Geometry check sheet. Reference: the model listing, model coordinates, mm. Face numbers are marked on the shaded views. A direction names the side the tool comes from. Give positions to 0.01 mm unless a question says otherwise; leave off trailing zeros. Order: outer loops, then holes, each group sorted by start corner. A loop starts at its lowest first (then second) coordinate and runs counter-clockwise, first axis right, second up. Notation, with made-up numbers: M 42,36.25 L 80,36.25 A24 cw 80,55.25 Z; hole C 28.5,-26 d3. An arc over 180 degrees is marked long. Put each result on its own line as item: value. Start each with the question number.
Q1. Material ranges on L1, parallel to X at y = -8.5, z = 19.5; L2, parallel to Z at x = -42, y = -15; L3, parallel to X at y = -1.5, z = 32.5, recorded low to high.
Q2. Section check A-A on z = 29.5. Record the cut outline in (x, y), then the cut area to 3 significant figures.
Q3. Go/stop test with flat-tipped pins: pin 1 (1 mm diameter, centred on x = -24.5, z = 7.5, fed in from +Y); pin 2 (11.5 mm diameter, centred on x = -35.5, z = 32.5, fed in from -Y); pin 3 (1.5 mm diameter, centred on x = -23.5, y = -32.5, fed in from +Z); pin 4 (19 mm diameter, centred on x = -27, y = -14.5, fed in from +Z). Record where each tip stops, or that it passes through.
Q4. Section check D-D on y = -21. Record the cut outline in (x, z).
Q5. Access from +Z, -Z, +X, -X, +Y, -Y to the whole of each face (thin tool, end or side, straight path). Record for the marked faces 1, 2 and 3.
Q6. Section check C-C on z = 14.5. Record the cut outline in (x, y).
Q7. Section check B-B on x = -10. Record the cut outline in (y, z), then the cut area to 3 significant figures.
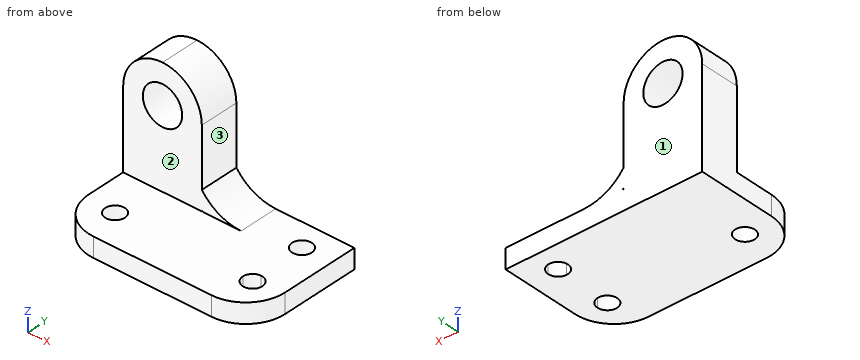
```python
from build123d import *

# Parameters (mm, degrees)
F1_DEPTH  = 38.1
F2_W      = 25.4
F2_H      = 38.1
F3_DEPTH  = 25.4
F4_R      = 6.35
F5_DEPTH  = 12.7
F7_DEPTH  = 6.35
F6_R      = 3.175
F8_DEPTH  = 6.35
F10_DEPTH = 12.7


with BuildPart() as f1:
    # F0 (on Front) → F1 (new body)
    with BuildSketch(Plane.XZ):
        Polygon((-37.0136184096, 45.1297735606), (-62.4136184096, 45.1297735606), (-62.4136184096, 0.6797735606), (1.0863815904, 0.6797735606), (1.0863815904, 7.0297735606), (-37.0136184096, 7.0297735606), align=None)
    extrude(amount=F1_DEPTH)

    # F2 (on face) → F3 (cut)
    with BuildSketch(Plane.XZ.offset(38.1)):
        with Locations((-49.7136184096, 26.0797735606)):
            Rectangle(F2_W, F2_H)
    extrude(amount=-F3_DEPTH, mode=Mode.SUBTRACT)

    # F4 (on face) → F5 (cut)
    with BuildSketch(Plane.XZ.offset(12.7)):
        with BuildLine():
            Line((-62.4136184096, 45.1297735606), (-62.4136184096, 32.4297735606))
            ThreePointArc((-62.4136184096, 32.4297735606), (-58.6938745306, 41.4100296816), (-49.7136184096, 45.1297735606))
            Line((-49.7136184096, 45.1297735606), (-62.4136184096, 45.1297735606))
        make_face()
        with BuildLine():
            Line((-37.0136184096, 45.1297735606), (-49.7136184096, 45.1297735606))
            ThreePointArc((-49.7136184096, 45.1297735606), (-40.7333622885, 41.4100296816), (-37.0136184096, 32.4297735606))
            Line((-37.0136184096, 32.4297735606), (-37.0136184096, 45.1297735606))
        make_face()
        with Locations((-49.7136184096, 32.4297735606)):
            Circle(F4_R)
    extrude(amount=-F5_DEPTH, mode=Mode.SUBTRACT)

    # F6 (on face) → F7 (cut)
    with BuildSketch(Plane.XY.offset(7.0297735606)):
        with BuildLine():
            Line((1.0863815904, -38.1), (1.0863815904, -25.4))
            ThreePointArc((1.0863815904, -25.4), (-2.6333622885, -34.3802561211), (-11.6136184096, -38.1))
            Line((-11.6136184096, -38.1), (1.0863815904, -38.1))
        make_face()
        with BuildLine():
            Line((-62.4136184096, -38.1), (-49.7136184096, -38.1))
            ThreePointArc((-49.7136184096, -38.1), (-58.6938745306, -34.3802561211), (-62.4136184096, -25.4))
            Line((-62.4136184096, -25.4), (-62.4136184096, -38.1))
        make_face()
    extrude(amount=-F7_DEPTH, mode=Mode.SUBTRACT)

    # F6 (on face) → F8 (cut)
    with BuildSketch(Plane.XY.offset(7.0297735606)):
        with BuildLine():
            ThreePointArc((-8.4208896913, -11.4911545114), (-6.2343188315, -10.5303998816), (-5.3360288183, -8.3174343067))
            ThreePointArc((-5.3360288183, -8.3174343067), (-10.7877388051, -6.1044687317), (-8.4208896913, -11.4911545114))
        make_face()
        with Locations((-52.429128431, -27.0451839786)):
            Circle(F6_R)
        with BuildLine():
            ThreePointArc((-4.804128431, -27.0451839786), (-5.7661628561, -24.7684739918), (-8.069267558, -23.8714637739))
            Line((-8.069267558, -23.8714637739), (-7.979128431, -27.0451839786))
            Line((-7.979128431, -27.0451839786), (-11.154128431, -27.0451839786))
            ThreePointArc((-11.154128431, -27.0451839786), (-7.979128431, -30.2201839786), (-4.804128431, -27.0451839786))
        make_face()
        with BuildLine():
            Line((-7.979128431, -27.0451839786), (-8.069267558, -23.8714637739))
            ThreePointArc((-8.069267558, -23.8714637739), (-10.2558384179, -24.8322184036), (-11.154128431, -27.0451839786))
            Line((-11.154128431, -27.0451839786), (-7.979128431, -27.0451839786))
        make_face()
    extrude(amount=-F8_DEPTH, mode=Mode.SUBTRACT)

    # F9 (on face) → F10 (join)
    with BuildSketch(Plane(origin=(0, 0, 0), x_dir=(-1, 0, 0), z_dir=(0, 1, 0))):
        with BuildLine():
            Line((37.0136184096, 7.5662416692), (37.0136184096, 13.3797735606))
            ThreePointArc((37.0136184096, 13.3797735606), (31.4131342381, 8.7057419035), (24.3136184096, 7.0297735606))
            Line((24.3136184096, 7.0297735606), (36.477150301, 7.0297735606))
            ThreePointArc((36.477150301, 7.0297735606), (36.8564905385, 7.1869014317), (37.0136184096, 7.5662416692))
        make_face()
    extrude(amount=-F10_DEPTH)


solid = f1.part
```
Results found:
1. L1: x = -62.41 to -37.01
1. L2: z = 0.68 to 7.03
1. L3: x = -62.41 to -56.06, -43.36 to -37.01
2. outline: M -62.41,-12.7 L -55.35,-12.7 L -55.35,0 L -62.41,0 Z; M -44.08,-12.7 L -37.01,-12.7 L -37.01,0 L -44.08,0 Z
2. area: 179 mm^2
3. pin 1: stops at y = 0
3. pin 2: stops at y = -12.7
3. pin 3: stops at z = 7.03
3. pin 4: stops at z = 12.53
4. outline: M -62.41,0.68 L 1.09,0.68 L 1.09,7.03 L -62.41,7.03 Z
5. face 1: +Z, -Z, +X, -X, +Y
5. face 2: +Z, +X, -X, -Y
5. face 3: +Z, +X, +Y, -Y
6. outline: M -62.41,-12.7 L -37.01,-12.7 L -37.01,0 L -62.41,0 Z
7. outline: M -38,0.68 L -29.49,0.68 L -29.49,7.03 L -38,7.03 Z; M -24.6,0.68 L -11.12,0.68 L -11.12,7.03 L -24.6,7.03 Z; M -5.51,0.68 L 0,0.68 L 0,7.03 L -5.51,7.03 Z
7. area: 175 mm^2
